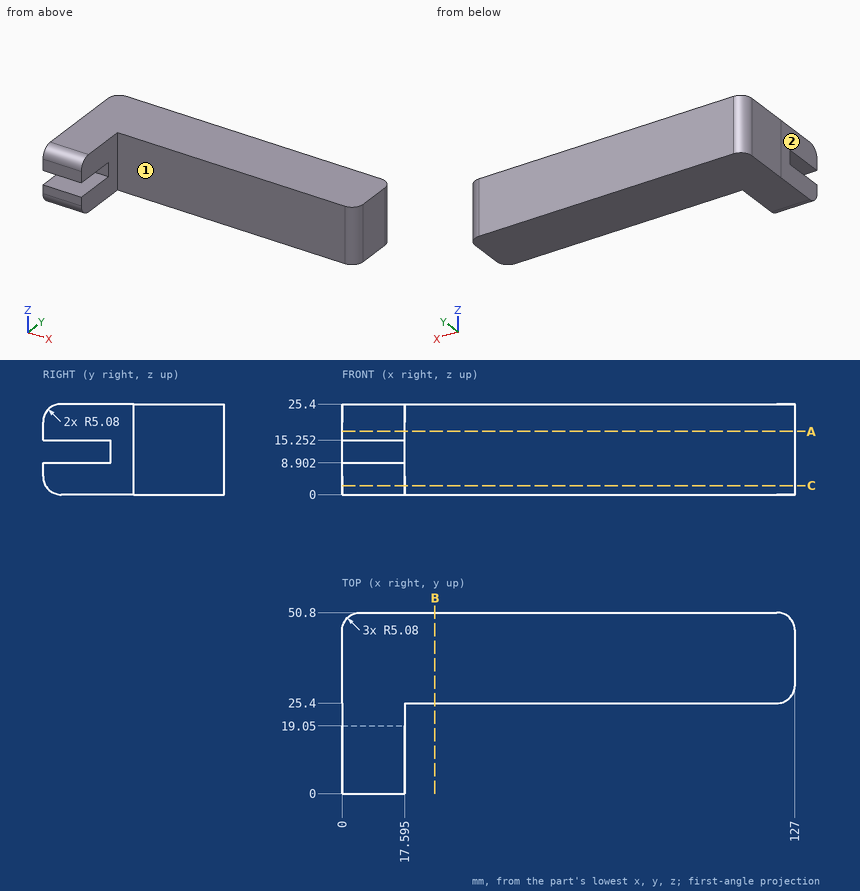
Answer from the drawing. Dimensions are ordinates in mm from the lowest x, y and z of the part. A direction names the side the tool comes from. Coordinates: 2 decimals unless noted, no trailing zeros. Write each loop counter-clockwise with the first axis right and the second up, starting at its lowest first coordinate (ties: lowest second). Pieces come first, ordered by that corner, then holes. Notation, with made-up numbers: (8.25, 63.25) -> (26.25, 63.25) arc R29 cw to (26.25, 88.25) -> close; hole circle Ø3 at (88.5, 63). An arc over 180 degrees is marked (long way). One line per question, with ' | ' between items.
1. Section B-B (x = 26) is taken. Determine the outline of the cut face in (y, z).
Verdict:
outline: (25.4, 0) -> (50.8, 0) -> (50.8, 25.4) -> (25.4, 25.4) -> close
2. Which of the six approach directions +Z, -Z, +X, -X, +Y, -Y give full straight-line access (tool end or side, diameter ignored) to the marked faces 1 and 2?
Verdict:
face 1: +Z, -Z, +X, -Y | face 2: +Z, -Z, -X, +Y, -Y
3. Given pin 1 Ø12.5 at (y, z) = (8, 17.5) entering from +X (1 decimal); pin 2 Ø7.5 at (x, z) = (53, 16.5) entering from -Y; pin 3 Ø1.9 at (x, z) = (8.5, 13) entering from -Y, each flat-ended and moving along its own axis, determine where each tip first touches the part or whether it passes through.
Verdict:
pin 1: stops at x = 17.6 | pin 2: stops at y = 25.4 | pin 3: stops at y = 19.05
4. Section A-A (z = 17.75) is taken. Determine the outline of the cut face in (x, y) (1 decimal).
Verdict:
outline: (0, 0) -> (17.6, 0) -> (17.6, 25.4) -> (121.9, 25.4) arc R5.1 ccw to (127, 30.5) -> (127, 45.7) arc R5.1 ccw to (121.9, 50.8) -> (5.1, 50.8) arc R5.1 ccw to (0, 45.7) -> close
5. Straight lines are drawn through the part: line 1 (X direction, y = 5.5, z = 19) (1 decimal); line 2 (Y direction, x = 106, z = 15); line 3 (Y direction, x = 12.5, z = 10.5). For each, find the intervals that lie inside material, in ascending order.
Verdict:
line 1: x = 0 to 17.6 | line 2: y = 25.4 to 50.8 | line 3: y = 19.05 to 50.8
6. Section C-C (z = 2.5) is taken. Determine the outline of the cut face in (x, y) (1 decimal).
Verdict:
outline: (0, 0.7) -> (17.6, 0.7) -> (17.6, 25.4) -> (121.9, 25.4) arc R5.1 ccw to (127, 30.5) -> (127, 45.7) arc R5.1 ccw to (121.9, 50.8) -> (5.1, 50.8) arc R5.1 ccw to (0, 45.7) -> close
